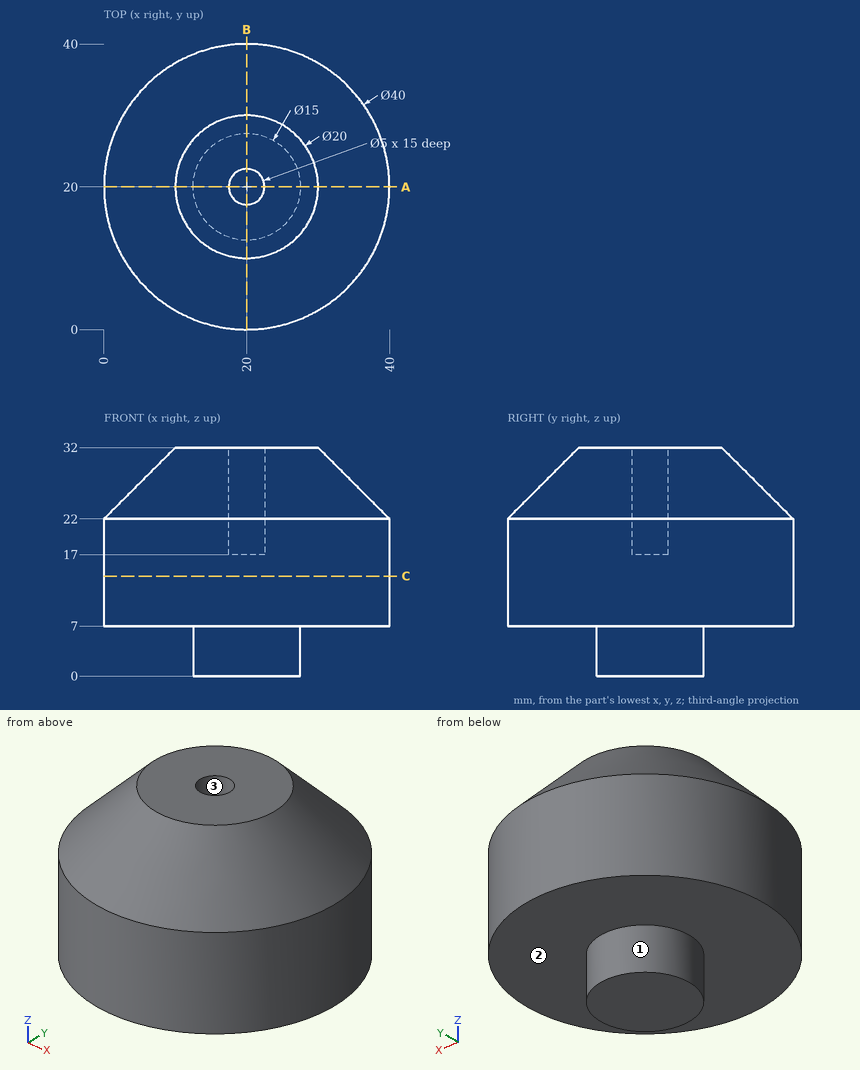
Design review of the part shown in the three views and the two pictorial views. Dimensions are in mm from the part's minimum x, y and z. Coordinates: 2 decimals unless noted, no trailing zeros. Order: outer loops, then holes, each group sorted by start corner. A loop starts at its lowest first (then second) coordinate and runs counter-clockwise, first axis right, second up.
1) Wall thickness on line 1 along Y through (x, z) = (20, 22); line 2 along Y through (x, z) = (20, 25); line 3 along X through (y, z) = (13, 14) (3 decimals): over which ranges is each line inside the solid? List them lowest first.
2) Take a section at A-A, the plane y = 20. Give the boundary of the cut face in (x, z).
3) Mouldability with a two-part tool opening along X and no side actions: class the marked faces 1, 2 and 3 as +X half, -X half, draft (parallel to the pull), parting line (faces both ways), or undercut.
4) Take a section at C-C, the plane z = 14. Give the boundary of the cut face in (x, y), and give its area (3 significant figures).
5) Clearance check with flat-ended pins moving along their axes: pin 1 (6 mm diameter, centred on y = 4.5, z = 21.5, fed in from -X); pin 2 (2 mm diameter, centred on y = 11, z = 12, fed in from -X); pin 3 (1 mm diameter, centred on y = 18, z = 20, fed in from +X); pin 4 (20 mm diameter, centred on x = 29.5, y = 24, fed in from -Z). State where each tip first meets the part, or that it passes through.
Returned:
1. line 1: y = 0 to 17.5, 22.5 to 40
1. line 2: y = 3 to 17.5, 22.5 to 37
1. line 3: x = 1.265 to 38.735
2. outline: (0, 7) - (12.5, 7) - (12.5, 0) - (27.5, 0) - (27.5, 7) - (40, 7) - (40, 22) - (30, 32) - (22.5, 32) - (22.5, 17) - (17.5, 17) - (17.5, 32) - (10, 32) - (0, 22) - close
3. face 1: parting line
3. face 2: draft
3. face 3: undercut
4. outline: circle Ø40 at (20, 20)
4. area: 1,260 mm2
5. pin 1: stops at x = 4.39
5. pin 2: stops at x = 1.67
5. pin 3: stops at x = 39.94
5. pin 4: stops at z = 0
